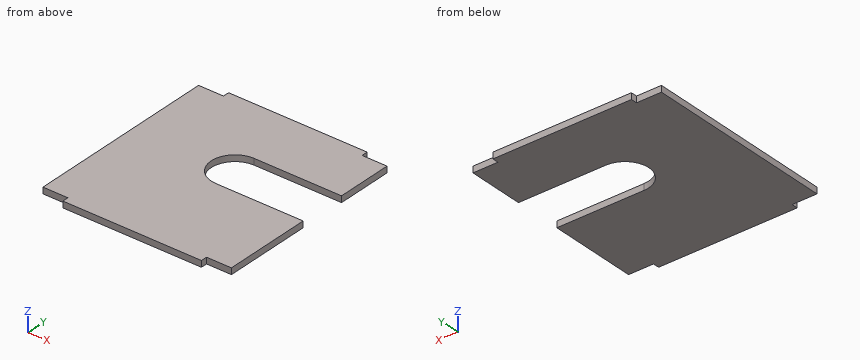
```python
from build123d import *

# Parameters (mm, degrees)
PAD_DEPTH = 2.5


with BuildPart() as part:
    # Sketch → Pad (new body, symmetric)
    with BuildSketch(Plane.XY):
        with BuildLine():
            Line((-55.5, 82), (-55.5, 77))
            Line((-55.5, 77), (-75.5, 77))
            Line((-75.5, 77), (-75.5, -77))
            Line((-75.5, -77), (-55.5, -77))
            Line((-55.5, -77), (-55.5, -82))
            Line((-55.5, -82), (55.5, -82))
            Line((55.5, -82), (55.5, -77))
            Line((55.5, -77), (75.5, -77))
            Line((75.5, -77), (75.5, -6))
            Line((75.5, -6), (5.5, -6))
            ThreePointArc((5.5, 32), (-13.5, 13), (5.5, -6))
            Line((5.5, 32), (75.5, 32))
            Line((75.5, 32), (75.5, 77))
            Line((75.5, 77), (55.5, 77))
            Line((55.5, 77), (55.5, 82))
            Line((55.5, 82), (-55.5, 82))
        make_face()
    extrude(amount=PAD_DEPTH, both=True)


solid = part.part
```
Source: CAD feature listing. Evaluate the final solid. Frame: model axes, mm. Coordinates: 2 decimals unless noted, no trailing zeros. Loops run counter-clockwise (first coordinate to the right, second up) from the corner with the lowest first, then second, coordinate; pieces in that order, holes last. Notation, with made-up numbers: M -3,33 L 44,33 A18 cw 44,59 Z; hole C -5,40 d4. An arc over 180 degrees is marked long. Use a Markdown table: item, result. Add a question column.
Q1. Section query A-A, the plane x = 43.5. Return loops of the section in (y, z), and give its area (3 significant figures).
Q2. Section query B-B, the plane z = 0.2. Return loops of the section in (x, y).
Q3. Material intervals for L1, parallel to Y at x = 48, z = 2.35; L2, parallel to Y at x = -64, z = -0.55; L3, parallel to Y at x = -7, z = -0.95, sorted ascending.
Q4. Section query C-C, the plane y = 13. Return loops of the section in (x, z).
Q5. Section query D-D, the plane x = -62.5. Return loops of the section in (y, z), and give its area (3 significant figures).
Q6. First-contact query: pin 1 (1.5 mm diameter, centred on x = -67, z = 0, fed in from -Y); pin 2 (2.5 mm diameter, centred on x = -63.5, z = -1, fed in from +Y); pin 3 (2.5 mm diameter, centred on y = 80.5, z = -0.5, fed in from +X). Flat tips, straight axial feed; report the tip coordinate or a pass-through.
Result:
| question | item | result |
|---|---|---|
| 1 | outline | M -82,-2.5 L -6,-2.5 L -6,2.5 L -82,2.5 Z; M 32,-2.5 L 82,-2.5 L 82,2.5 L 32,2.5 Z |
| 1 | area | 630 mm2 |
| 2 | outline | M -75.5,-77 L -55.5,-77 L -55.5,-82 L 55.5,-82 L 55.5,-77 L 75.5,-77 L 75.5,-6 L 5.5,-6 A19 cw 5.5,32 L 75.5,32 L 75.5,77 L 55.5,77 L 55.5,82 L -55.5,82 L -55.5,77 L -75.5,77 Z |
| 3 | L1 | y = -82 to -6, 32 to 82 |
| 3 | L2 | y = -77 to 77 |
| 3 | L3 | y = -82 to -1.31, 27.31 to 82 |
| 4 | outline | M -75.5,-2.5 L -13.5,-2.5 L -13.5,2.5 L -75.5,2.5 Z |
| 5 | outline | M -77,-2.5 L 77,-2.5 L 77,2.5 L -77,2.5 Z |
| 5 | area | 770 mm2 |
| 6 | pin 1 | stops at y = -77 |
| 6 | pin 2 | stops at y = 77 |
| 6 | pin 3 | stops at x = 55.5 |
